```python
from build123d import *

# Parameters (mm, degrees)
SKETCH1_R           = 49.5046
BOSS_EXTRUDE1_DEPTH = 5.08
SKETCH2_R           = 47.625
BOSS_EXTRUDE2_DEPTH = 3.175
SKETCH3_R           = 6.35
SKETCH3_R_2         = 3.96875
SKETCH3_R_3         = 3.175
CUT_EXTRUDE1_DEPTH  = 9.255
SKETCH4_R           = 53.657769874
CUT_EXTRUDE2_DEPTH  = 3.175


with BuildPart() as part:
    # Sketch1 → Boss-Extrude1 (new body)
    with BuildSketch(Plane.XY):
        Circle(SKETCH1_R)
    extrude(amount=BOSS_EXTRUDE1_DEPTH)

    # Sketch2 → Boss-Extrude2 (add)
    with BuildSketch(Plane.XY.offset(5.08)):
        Circle(SKETCH2_R)
    extrude(amount=BOSS_EXTRUDE2_DEPTH)

    # Sketch3 → Cut-Extrude1 (cut, through all)
    with BuildSketch(Plane.XY.offset(8.255)):
        with Locations((-12.7, -31.166793627)):
            Circle(SKETCH3_R)
        with Locations((12.7, -31.166793627)):
            Circle(SKETCH3_R)
        with Locations((-36.83, 0)):
            Circle(SKETCH3_R_2)
        with Locations((36.83, 0)):
            Circle(SKETCH3_R_2)
        with Locations((-14.921345457, -10.968575281)):
            Circle(SKETCH3_R_3)
    extrude(amount=-CUT_EXTRUDE1_DEPTH, mode=Mode.SUBTRACT)

    # Sketch4 → Cut-Extrude2 (cut)
    with BuildSketch(Plane.XY.offset(8.255)):
        Circle(SKETCH4_R)
    extrude(amount=-CUT_EXTRUDE2_DEPTH, mode=Mode.SUBTRACT)


solid = part.part
```
Check sheet for the modelled part. Datum: model origin and axes. Units: mm. Coordinates: 2 decimals unless noted, no trailing zeros. Write each loop counter-clockwise with the first axis right and the second up, starting at its lowest first coordinate (ties: lowest second). Pieces come first, ordered by that corner, then holes. Notation, with made-up numbers: M -12.75,-8 L 1.25,-8 A28 cw 1.25,30 Z; hole C -3,28 d4. An arc over 180 degrees is marked long. Use one line per item in the form item = value.
Item 1: Sectioned sample at B-B, the plane x = 12.7. Record the cut outline in (y, z), and give its area (3 significant figures).
Answer below:
outline = M -47.85,0 L -37.52,0 L -37.52,5.08 L -47.85,5.08 Z; M -24.82,0 L 47.85,0 L 47.85,5.08 L -24.82,5.08 Z
area = 422 mm^2
Item 2: Sectioned sample at D-D, the plane x = 36.83. Record the cut outline in (y, z), and give its area (3 significant figures).
Answer below:
outline = M -33.08,0 L -3.97,0 L -3.97,5.08 L -33.08,5.08 Z; M 3.97,0 L 33.08,0 L 33.08,5.08 L 3.97,5.08 Z
area = 296 mm^2
Item 3: Sectioned sample at C-C, the plane z = 2. State how many separate pieces and enclosed holes the cut face has, and give its area (3 significant figures).
Answer below:
separate_pieces = 1
enclosed_holes = 5
area = 7,320 mm^2
Item 4: Release check for a two-part mould opening along Y. For faces 1 (the face through (-11.988, -12.185, 2.576)), 2 (the face through (-6.445, 49.083, 2.504)), 3 (the face through (-1, 1, 0)) record: pulls with the +Y half, pulls with the -Y half, needs draft (parallel to the pull), parting line crosses it, or undercut.
Answer below:
face_1 = undercut
face_2 = parting line crosses it
face_3 = needs draft
Item 5: Sectioned sample at A-A, the plane y = 0. Record the cut outline in (x, z), and give its area (3 significant figures).
Answer below:
outline = M -49.5,0 L -40.8,0 L -40.8,5.08 L -49.5,5.08 Z; M -32.86,0 L 32.86,0 L 32.86,5.08 L -32.86,5.08 Z; M 40.8,0 L 49.5,0 L 49.5,5.08 L 40.8,5.08 Z
area = 422 mm^2
Item 6: Material ranges on L1, parallel to Y at x = 37, z = 0.4; L2, parallel to Y at x = -16.5, z = 1.75; L3, parallel to Y at x = -40, z = 1.85, recorded low to high. Write a range as from..to.
Answer below:
L1 = -32.89..-3.97, 3.97..32.89
L2 = -46.67..-36.25, -26.08..-13.72, -8.21..46.67
L3 = -29.17..-2.39, 2.39..29.17
